Work out the finished part from the listing and answer in its coordinate system (mm). A direction names the side the tool comes from. Round coordinates to 2 decimals unless told otherwise and drop trailing zeros. Write each loop counter-clockwise with the first axis right and the second up, starting at its lowest first coordinate (ties: lowest second). Pieces come first, ordered by that corner, then holes. Notation, with made-up numbers: (47, -35.75) -> (80, -35.75) arc R21 ccw to (80, -16.75) -> close; hole circle Ø5 at (29, 89.25). An arc over 180 degrees is marked (long way). One line per item, written item: value.
```python
from build123d import *

# Parameters (mm, degrees)
EXTRUDE_THIN1_DEPTH = 76.2
FILLET1_R           = 6.35
SKETCH3_R           = 5.470235349
CUT_EXTRUDE2_DEPTH  = 76.2
FILLET2_R           = 3.175


with BuildPart() as part:
    # Sketch1 → Extrude-Thin1 (new body)
    with BuildSketch(Plane(origin=(0, 0, 0), x_dir=(0, 0, -1), z_dir=(1, 0, 0))):
        Polygon((74.026491926, 0), (0, 0), (0, 50.8), (6.35, 50.8), (6.35, 6.35), (74.026491926, 6.35), align=None)
    extrude(amount=EXTRUDE_THIN1_DEPTH)

    # Fillet1
    fillet1_edges = [part.edges().sort_by_distance(p)[0] for p in [
        (76.2, 3.175, -74.026491926),
        (0, 3.175, -74.026491926),
        (0, 50.8, -3.175),
        (76.2, 50.8, -3.175),
    ]]
    fillet(fillet1_edges, radius=FILLET1_R)

    # Sketch3 → Cut-Extrude2 (cut)
    with BuildSketch(Plane.XY):
        with Locations((12.201854518, 38.1)):
            Circle(SKETCH3_R)
        with Locations((63.998145482, 38.1)):
            Circle(SKETCH3_R)
    extrude(amount=-CUT_EXTRUDE2_DEPTH, mode=Mode.SUBTRACT)

    # Fillet2
    fillet2_edges = [part.edges().sort_by_distance(p)[0] for p in [
        (38.1, 6.35, -6.35),
    ]]
    fillet(fillet2_edges, radius=FILLET2_R)


solid = part.part
```
(1) For a pull along Y with two mould halves and no side action, classify faces 3 (the face through (38, 30, -6.35)), 4 (the face through (69.05, 36, -3.13)), 5 (the face through (38.63, 7.26, -7.3)), 6 (the face through (38, 0, -38)) as pulls with the +Y half, pulls with the -Y half, needs draft (parallel to the pull), parting line crosses it, or undercut.
Reported:
face 3: needs draft
face 4: undercut
face 5: pulls with the +Y half
face 6: pulls with the -Y half
(2) Find section D-D on z = -23. Give the vertices of the cut face in (x, y).
Reported:
outline: (0, 0) -> (76.2, 0) -> (76.2, 6.35) -> (0, 6.35) -> close
(3) Flat-ended cylindrical pins translate along their axes: pin 1 Ø8 at (x, y) = (20, 39) entering from -Z; pin 2 Ø12 at (x, y) = (38.5, 40) entering from +Z; pin 3 Ø12 at (x, z) = (10.5, -44) entering from +Y. Find the tip coordinate at first contact, or state that the pin passes through.
Reported:
pin 1: stops at z = -6.35
pin 2: stops at z = 0
pin 3: stops at y = 6.35
(4) Consider probe 1 along X at (y, z) = (38, -1); probe 2 along Y at (x, z) = (44.5, -43.5). Determine where each line is inside the solid, lowest interval first.
Reported:
probe 1: x = 0 to 6.73, 17.67 to 58.53, 69.47 to 76.2
probe 2: y = 0 to 6.35
(5) Find section A-A on y = 38.1. Give the vertices of the cut face in (x, z), plus the area to 3 significant figures.
Reported:
outline: (0, -6.35) -> (6.73, -6.35) -> (6.73, 0) -> (0, 0) -> close; (17.67, -6.35) -> (58.53, -6.35) -> (58.53, 0) -> (17.67, 0) -> close; (69.47, -6.35) -> (76.2, -6.35) -> (76.2, 0) -> (69.47, 0) -> close
area: 345 mm2
(6) A tool of negligible diameter and unlimited length cuts with its end or side. For faces 1 (the face through (76.2, 6, -26)), 2 (the face through (38, 6.35, -41)), from which of +Z, -Z, +X, -X, +Y, -Y can it reach the whole face along a straight path? Write none if from no direction.
Reported:
face 1: +Z, -Z, +X, +Y, -Y
face 2: -Z, +X, -X, +Y
